Geometry check sheet. Reference: the model listing, model coordinates, mm. Coordinates: 2 decimals unless noted, no trailing zeros. Write each loop counter-clockwise with the first axis right and the second up, starting at its lowest first coordinate (ties: lowest second). Pieces come first, ordered by that corner, then holes.
from build123d import *

# Parameters (mm, degrees)
SKIZZE1_R                       = 2.15
AUFSATZ_LINEAR_AUSTRAGEN1_DEPTH = 104


with BuildPart() as part:
    # Skizze1 → Aufsatz-Linear austragen1 (new body)
    with BuildSketch(Plane.XY.offset(100)):
        with BuildLine():
            Line((12.499999989, 1.499999999), (12.499999989, 0.800000002))
            ThreePointArc((12.499999989, 0.800000002), (12.734314564, 0.234314576), (13.299999991, 0))
            Line((13.299999991, 0), (18, 0))
            ThreePointArc((18, 0), (19.414213562, 0.585786438), (20, 2))
            Line((20, 2), (20, 6.700000003))
            ThreePointArc((20, 6.700000003), (19.765685425, 7.265685427), (19.2, 7.500000003))
            Line((19.2, 7.500000003), (18.499999995, 7.500000003))
            ThreePointArc((18.499999995, 7.500000003), (18.287867961, 7.412132037), (18.199999995, 7.200000003))
            Line((18.199999995, 7.200000003), (18.199999995, 5.082411607))
            ThreePointArc((18.199999995, 5.082411607), (17.686138517, 4.313363558), (16.778984491, 4.493807713))
            Line((16.778984491, 4.493807713), (14.528679651, 6.744112553))
            ThreePointArc((14.528679651, 6.744112553), (13.878361397, 7.717382599), (13.649999995, 8.865432896))
            Line((13.649999995, 8.865432896), (13.649999995, 11.134567106))
            ThreePointArc((13.649999995, 11.134567106), (13.878361397, 12.282617403), (14.528679651, 13.255887449))
            Line((14.528679651, 13.255887449), (16.778984493, 15.506192291))
            ThreePointArc((16.778984493, 15.506192291), (17.686138518, 15.686636446), (18.199999995, 14.917588398))
            Line((18.199999995, 14.917588398), (18.199999995, 12.800000001))
            ThreePointArc((18.199999995, 12.800000001), (18.287867961, 12.587867966), (18.499999996, 12.5))
            Line((18.499999996, 12.5), (19.199999998, 12.5))
            ThreePointArc((19.199999998, 12.5), (19.765685424, 12.734314576), (20, 13.300000003))
            Line((20, 13.300000003), (20, 18))
            ThreePointArc((20, 18), (19.414213562, 19.414213562), (18, 20))
            Line((18, 20), (13.299999989, 20))
            ThreePointArc((13.299999989, 20), (12.734314564, 19.765685425), (12.499999989, 19.2))
            Line((12.499999989, 19.2), (12.499999989, 18.499999999))
            ThreePointArc((12.499999989, 18.499999999), (12.587867954, 18.287867964), (12.799999989, 18.199999999))
            Line((12.799999989, 18.199999999), (14.917588395, 18.199999999))
            ThreePointArc((14.917588395, 18.199999999), (15.686636445, 17.68613852), (15.50619229, 16.778984493))
            Line((15.50619229, 16.778984493), (13.255887454, 14.528679658))
            ThreePointArc((13.255887454, 14.528679658), (12.282617408, 13.878361404), (11.134567111, 13.650000002))
            Line((11.134567111, 13.650000002), (8.865432888, 13.650000002))
            ThreePointArc((8.865432888, 13.650000002), (7.717382592, 13.878361404), (6.744112546, 14.528679658))
            Line((6.744112546, 14.528679658), (4.493807706, 16.778984498))
            ThreePointArc((4.493807706, 16.778984498), (4.313363551, 17.686138522), (5.082411599, 18.199999999))
            Line((5.082411599, 18.199999999), (7.199999999, 18.199999999))
            ThreePointArc((7.199999999, 18.199999999), (7.412132034, 18.287867965), (7.5, 18.5))
            Line((7.5, 18.5), (7.5, 19.199999998))
            ThreePointArc((7.5, 19.199999998), (7.265685424, 19.765685424), (6.699999997, 20))
            Line((6.699999997, 20), (2, 20))
            ThreePointArc((2, 20), (0.585786438, 19.414213562), (0, 18))
            Line((0, 18), (0, 13.3))
            ThreePointArc((0, 13.3), (0.234314575, 12.734314575), (0.8, 12.5))
            Line((0.8, 12.5), (1.500000004, 12.5))
            ThreePointArc((1.500000004, 12.5), (1.712132038, 12.587867966), (1.800000004, 12.8))
            Line((1.800000004, 12.8), (1.800000004, 14.917588391))
            ThreePointArc((1.800000004, 14.917588391), (2.313861482, 15.68663644), (3.221015508, 15.506192285))
            Line((3.221015508, 15.506192285), (5.471320345, 13.255887449))
            ThreePointArc((5.471320345, 13.255887449), (6.121638599, 12.282617402), (6.350000001, 11.134567106))
            Line((6.350000001, 11.134567106), (6.350000001, 8.865432891))
            ThreePointArc((6.350000001, 8.865432891), (6.121638599, 7.717382594), (5.471320345, 6.744112548))
            Line((5.471320345, 6.744112548), (3.221015505, 4.493807708))
            ThreePointArc((3.221015505, 4.493807708), (2.313861481, 4.313363554), (1.800000004, 5.082411601))
            Line((1.800000004, 5.082411601), (1.800000004, 7.200000001))
            ThreePointArc((1.800000004, 7.200000001), (1.712132038, 7.412132036), (1.500000003, 7.500000002))
            Line((1.500000003, 7.500000002), (0.800000003, 7.500000002))
            ThreePointArc((0.800000003, 7.500000002), (0.234314576, 7.265685427), (0, 6.7))
            Line((0, 6.7), (0, 2))
            ThreePointArc((0, 2), (0.585786438, 0.585786438), (2, 0))
            Line((2, 0), (6.7, 0))
            ThreePointArc((6.7, 0), (7.265685425, 0.234314575), (7.5, 0.8))
            Line((7.5, 0.8), (7.5, 1.5))
            ThreePointArc((7.5, 1.5), (7.412132034, 1.712132034), (7.2, 1.8))
            Line((7.2, 1.8), (5.0824116, 1.8))
            ThreePointArc((5.0824116, 1.8), (4.313363551, 2.313861478), (4.493807706, 3.221015504))
            Line((4.493807706, 3.221015504), (6.744112546, 5.471320344))
            ThreePointArc((6.744112546, 5.471320344), (7.717382592, 6.121638598), (8.865432889, 6.35))
            Line((8.865432889, 6.35), (11.134567106, 6.35))
            ThreePointArc((11.134567106, 6.35), (12.282617403, 6.121638598), (13.255887449, 5.471320344))
            Line((13.255887449, 5.471320344), (15.506192291, 3.221015502))
            ThreePointArc((15.506192291, 3.221015502), (15.686636446, 2.313861477), (14.917588398, 1.8))
            Line((14.917588398, 1.8), (12.79999999, 1.8))
            ThreePointArc((12.79999999, 1.8), (12.587867955, 1.712132034), (12.499999989, 1.499999999))
        make_face()
        with Locations((10, 10)):
            Circle(SKIZZE1_R, mode=Mode.SUBTRACT)
    extrude(amount=-AUFSATZ_LINEAR_AUSTRAGEN1_DEPTH)


solid = part.part
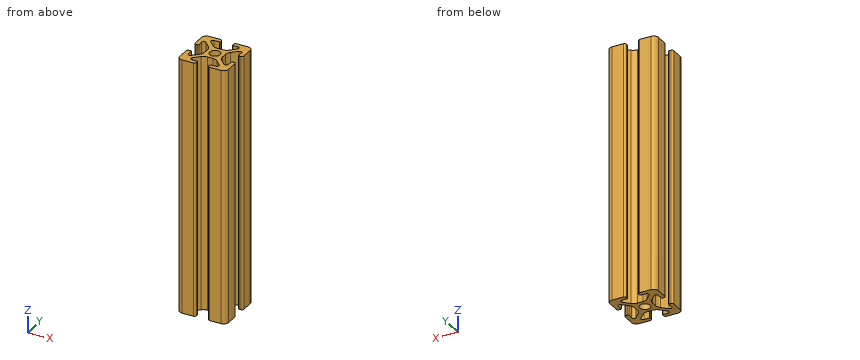
1. Thickness scan on line 1 along Y through (x, z) = (10, 28.5); line 2 along Y through (x, z) = (17.5, 75); line 3 along Y through (x, z) = (6.75, 22). Record the ranges inside material, lowest first.
Computed values:
line 1: y = 6.35 to 7.85, 12.15 to 13.65
line 2: y = 0 to 4.26, 15.74 to 20
line 3: y = 0 to 1.8, 5.48 to 14.52, 18.2 to 20
2. Gauge pin test, flat ends, axial feed: pin 1 Ø0.7 at (y, z) = (10, 70.5) entering from -X; pin 2 Ø1.1 at (x, z) = (10, 62) entering from -Y; pin 3 Ø2.5 at (x, z) = (10, 59.5) entering from +Y. Record the tip position at first contact, or that the pin passes through.
Computed values:
pin 1: stops at x = 6.35
pin 2: stops at y = 6.35
pin 3: stops at y = 13.65
3. Sectioned sample at A-A, the plane x = 10. Record the boundary of the cut face in (y, z), and give its area (3 significant figures).
Computed values:
outline: (6.35, -4) - (7.85, -4) - (7.85, 100) - (6.35, 100) - close; (12.15, -4) - (13.65, -4) - (13.65, 100) - (12.15, 100) - close
area: 312 mm2
